Design review of the part built by this model. Coordinates are the model's own, in mm. A direction names the side the tool comes from. Coordinates: 2 decimals unless noted, no trailing zeros. Order: outer loops, then holes, each group sorted by start corner. A loop starts at its lowest first (then second) coordinate and runs counter-clockwise, first axis right, second up. Notation, with made-up numbers: (-16, 5) -> (41, 5) arc R29 cw to (41, 43) -> close; hole circle Ø1 at (66.5, 60.25). An arc over 180 degrees is marked (long way). Use a Markdown table: item, result. Add a question column.
Q1. Machinability: for faces 1 (the face through (0, 2.796, 0)), 2 (the face through (0, 27.436, -4)), 3 (the face through (0.81, 8.38, -3.64)), which of the approach directions +Z, -Z, +X, -X, +Y, -Y give a long, thin tool a straight path to every point of the face, cutting with its end or side? Answer none if there is none.
Q2. Add section A-A (y = 35). State the section outline as (x, z) points, then the cut area to 3 significant figures.
Q3. Wall thickness on probe 1 along Y at (x, z) = (5.75, -6); probe 2 along Y at (x, z) = (11, 5.75); probe 3 along X at (y, z) = (19.5, -7.75): over which ranges is each line inside the solid? List them lowest first.
Q4. Insertion check: pin 1 (6 mm diameter, centred on y = 26.5, z = 9, fed in from +X); pin 2 (8 mm diameter, centred on x = 7.5, y = 28, fed in from +Z); pin 3 (8 mm diameter, centred on x = -7.5, z = 5.5, fed in from -Y). Each pin has a flat end and moves straight along its axis. Give the tip position at first contact, or say it passes through.
from build123d import *


with BuildPart() as part:
    # Эскиз1 → Повернуть1 (revolve)
    with BuildSketch(Plane.XY):
        with BuildLine():
            Line((0, 42.221330192), (-3, 42.221330192))
            Line((-3, 42.221330192), (-3, 32.221330192))
            Line((-3, 32.221330192), (-3.728781423, 32.221330192))
            Line((-3.728781423, 32.221330192), (-3.728781423, 27.435605162))
            Line((-3.728781423, 27.435605162), (-5.773927938, 27.435605162))
            ThreePointArc((-5.773927938, 27.435605162), (-14.185723229, 19.023809872), (-5.773927938, 10.612014581))
            Line((-5.773927938, 10.612014581), (-3.728781423, 10.612014581))
            Line((-3.728781423, 10.612014581), (-3.728781423, 6.218549743))
            Line((-3.728781423, 6.218549743), (-3, 6.218549743))
            Line((-3, 6.218549743), (-3, 2.795657314))
            Line((-3, 2.795657314), (0, 2.795657314))
            Line((0, 2.795657314), (0, 42.221330192))
        make_face()
    revolve(axis=Axis((0, 0, 0), (0, 1, 0)))


solid = part.part
Established:
| question | item | result |
|---|---|---|
| 1 | face 1 | +Z, -Z, +X, -X, -Y |
| 1 | face 2 | +Y |
| 1 | face 3 | -Y |
| 2 | outline | circle Ø6 at (0, 0) |
| 2 | area | 28.3 mm^2 |
| 3 | probe 1 | 11 to 27.04 |
| 3 | probe 2 | 13.86 to 24.19 |
| 3 | probe 3 | -11.87 to 11.87 |
| 4 | pin 1 | x = 10.2 |
| 4 | pin 2 | z = 10.81 |
| 4 | pin 3 | y = 10.61 |
